Geometry check sheet. Reference: the model listing, model coordinates, mm. Give positions to 0.01 mm unless a question says otherwise; leave off trailing zeros. Write each loop counter-clockwise with the first axis right and the second up, starting at its lowest first coordinate (ties: lowest second). Pieces come first, ordered by that corner, then holes.
(1) Cross-section at A-A (y = 0). Record the boundary of the cut face in (x, z), and give its area (3 significant figures).
(2) Depth check by flat-ended pin: P1, Ø12, axis at x = 13.5, y = -5.5, coming from the -Z side. Enter the tip coordinate at first touch or a pass-through.
(3) Cross-section at C-C (z = 1.3). Count the separate pieces of the cut face and the enclosed holes in it, and give its area (3 significant figures).
(4) Cross-section at B-B (x = -17). Record the boundary of the cut face in (y, z).
(5) Thickness scan on line 1 along Y through (x, z) = (0, 1.2); line 2 along Y through (x, z) = (8.5, 0.9); line 3 along Y through (x, z) = (0.5, 0.7). Record the ranges inside material, lowest first.
(6) Cross-section at D-D (y = -6.25). Record the boundary of the cut face in (x, z).
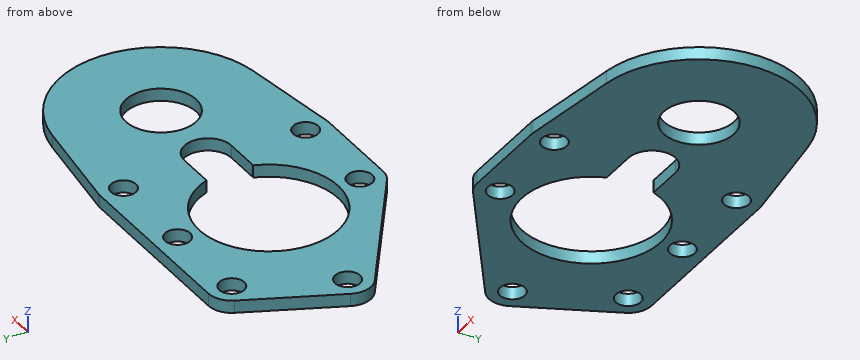
```python
from build123d import *

# Parameters (mm, degrees)
SKETCH1_R           = 3
SKETCH1_R_2         = 4.5
SKETCH1_R_3         = 1.6
BOSS_EXTRUDE3_DEPTH = 1.6
CUT_EXTRUDE1_DEPTH  = 10
SKETCH3_R           = 8.9
CUT_EXTRUDE2_DEPTH  = 30


with BuildPart() as part:
    # Sketch1 → Boss-Extrude3 (new body)
    with BuildSketch(Plane.XY):
        with BuildLine():
            Line((12.073070054, 14.639688463), (24.958502044, 12.880515151))
            ThreePointArc((24.958502044, 12.880515151), (36.2, 0), (24.958502044, -12.880515151))
            Line((24.958502044, -12.880515151), (12.073070054, -14.639688463))
            ThreePointArc((12.073070054, -14.639688463), (11.870633815, -14.660360595), (11.66726189, -14.66726189))
            Line((11.66726189, -14.66726189), (0, -14.66726189))
            ThreePointArc((0, -14.66726189), (-0.888679088, -14.53261518), (-1.697586366, -14.140761542))
            Line((-1.697586366, -14.140761542), (-18.697586366, -2.473499652))
            ThreePointArc((-18.697586366, -2.473499652), (-19.891071988, -0.801063519), (-19.728500117, 1.247111507))
            Line((-19.728500117, 1.247111507), (-14.395762007, 12.914373397))
            ThreePointArc((-14.395762007, 12.914373397), (-13.288783625, 14.191279968), (-11.66726189, 14.66726189))
            Line((-11.66726189, 14.66726189), (11.66726189, 14.66726189))
            ThreePointArc((11.66726189, 14.66726189), (11.870633815, 14.660360595), (12.073070054, 14.639688463))
        make_face()
        Circle(SKETCH1_R, mode=Mode.SUBTRACT)
        with Locations((23.2, 0)):
            Circle(SKETCH1_R_2, mode=Mode.SUBTRACT)
        with Locations((8.6, 0)):
            Circle(SKETCH1_R, mode=Mode.SUBTRACT)
        with Locations((-17, 0)):
            Circle(SKETCH1_R_3, mode=Mode.SUBTRACT)
        with Locations((0, -11.66726189)):
            Circle(SKETCH1_R_3, mode=Mode.SUBTRACT)
        with Locations((11.66726189, -11.66726189)):
            Circle(SKETCH1_R_3, mode=Mode.SUBTRACT)
        with Locations((-11.66726189, 11.66726189)):
            Circle(SKETCH1_R_3, mode=Mode.SUBTRACT)
        with Locations((0, 11.66726189)):
            Circle(SKETCH1_R_3, mode=Mode.SUBTRACT)
        with Locations((11.66726189, 11.66726189)):
            Circle(SKETCH1_R_3, mode=Mode.SUBTRACT)
    extrude(amount=BOSS_EXTRUDE3_DEPTH)

    # Sketch2 → Cut-Extrude1 (cut)
    with BuildSketch(Plane.XY.offset(1.6)):
        with BuildLine():
            Line((8.6, 3), (13.1, 3))
            ThreePointArc((13.1, 3), (16.1, 0), (13.1, -3))
            Line((13.1, -3), (8.6, -3))
            ThreePointArc((8.6, -3), (5.6, 0), (8.6, 3))
        make_face()
    extrude(amount=-CUT_EXTRUDE1_DEPTH, mode=Mode.SUBTRACT)

    # Sketch3 → Cut-Extrude2 (cut)
    with BuildSketch(Plane.XY.offset(1.6)):
        Circle(SKETCH3_R)
    extrude(amount=-CUT_EXTRUDE2_DEPTH, mode=Mode.SUBTRACT)


solid = part.part
```
Reply:
1. outline: (-20, 0) - (-18.6, 0) - (-18.6, 1.6) - (-20, 1.6) - close; (-15.4, 0) - (-8.9, 0) - (-8.9, 1.6) - (-15.4, 1.6) - close; (16.1, 0) - (18.7, 0) - (18.7, 1.6) - (16.1, 1.6) - close; (27.7, 0) - (36.2, 0) - (36.2, 1.6) - (27.7, 1.6) - close
1. area: 30.4 mm2
2. P1: stops at z = 0
3. separate pieces: 1
3. enclosed holes: 8
3. area: 943 mm2
4. outline: (-3.64, 0) - (-1.6, 0) - (-1.6, 1.6) - (-3.64, 1.6) - close; (1.6, 0) - (7.22, 0) - (7.22, 1.6) - (1.6, 1.6) - close
5. line 1: y = -14.67 to -13.27, -10.07 to -8.9, 8.9 to 10.07, 13.27 to 14.67
5. line 2: y = -14.67 to -3, 3 to 14.67
5. line 3: y = -14.67 to -13.19, -10.15 to -8.89, 8.89 to 10.15, 13.19 to 14.67
6. outline: (-13.19, 0) - (-6.34, 0) - (-6.34, 1.6) - (-13.19, 1.6) - close; (6.34, 0) - (34.6, 0) - (34.6, 1.6) - (6.34, 1.6) - close
